from build123d import *

# Parameters (mm, degrees)
F0_R     = 11.2476084484
F1_DEPTH = 14.478


# Not quite as in the source:
# - a feature of the source that left no trace in its solid (it failed there, or was rolled back) is left out


with BuildPart() as f1:
    # F0 (on Top) → F1 (new body)
    with BuildSketch(Plane.XY):
        Polygon((13.876531439, -13.876531439), (19.6243789597, 0), (13.876531439, 13.876531439), (0, 19.6243789597), (-13.876531439, 13.876531439), (-19.6243789597, 0), (-13.876531439, -13.876531439), (0, -19.6243789597), align=None)
        Circle(F0_R, mode=Mode.SUBTRACT)
        Circle(F0_R)
    extrude(amount=F1_DEPTH)


solid = f1.part
Design review of the part built by this model. Coordinates are the model's own, in mm. Coordinates: 2 decimals unless noted, no trailing zeros. Order: outer loops, then holes, each group sorted by start corner. A loop starts at its lowest first (then second) coordinate and runs counter-clockwise, first axis right, second up. Notation, with made-up numbers: (-16, 61.5) -> (-8, 61.5) arc R31 ccw to (-8, 98.5) -> close; hole circle Ø3 at (-1, -13). An arc over 180 degrees is marked (long way). Use one line per item in the form item = value. Start each with the question number.
(1) Insertion check: pin 1 (1 mm diameter, centred on x = 9.5, y = 9, fed in from -Z); pin 2 (3 mm diameter, centred on y = 3.5, z = 12.5, fed in from +X); pin 3 (5 mm diameter, centred on y = 9, z = 8, fed in from +X); pin 4 (6 mm diameter, centred on y = 13.5, z = 12, fed in from -X). Each pin has a flat end and moves straight along its axis. Give the tip position at first contact, or say it passes through.
(2) Add section C-C on y = 10.5. State the section outline as (x, z) points.
(3) For probe 1 along X at (y, z) = (18.5, 10.25); probe 2 along X at (y, z) = (-9.5, 1.75); probe 3 along Y at (x, z) = (-12, 5), list the stretches that pass through material, from the lowest coordinate up.
(4) Add section A-A on z = 3.25. State the section outline as (x, y) points, plus the area to 3 significant figures.
(5) Add section B-B on x = 9. State the section outline as (y, z) points.
Answer block:
q1.pin_1 = 0
q1.pin_2 = 18.8
q1.pin_3 = 16.93
q1.pin_4 = -15.28
q2.outline = (-15.28, 0) -> (15.28, 0) -> (15.28, 14.48) -> (-15.28, 14.48) -> close
q3.probe_1 = -2.71 to 2.71
q3.probe_2 = -15.69 to 15.69
q3.probe_3 = -14.65 to 14.65
q4.outline = (-19.62, 0) -> (-13.88, -13.88) -> (0, -19.62) -> (13.88, -13.88) -> (19.62, 0) -> (13.88, 13.88) -> (0, 19.62) -> (-13.88, 13.88) -> close
q4.area = 1,090 mm²
q5.outline = (-15.9, 0) -> (15.9, 0) -> (15.9, 14.48) -> (-15.9, 14.48) -> close
